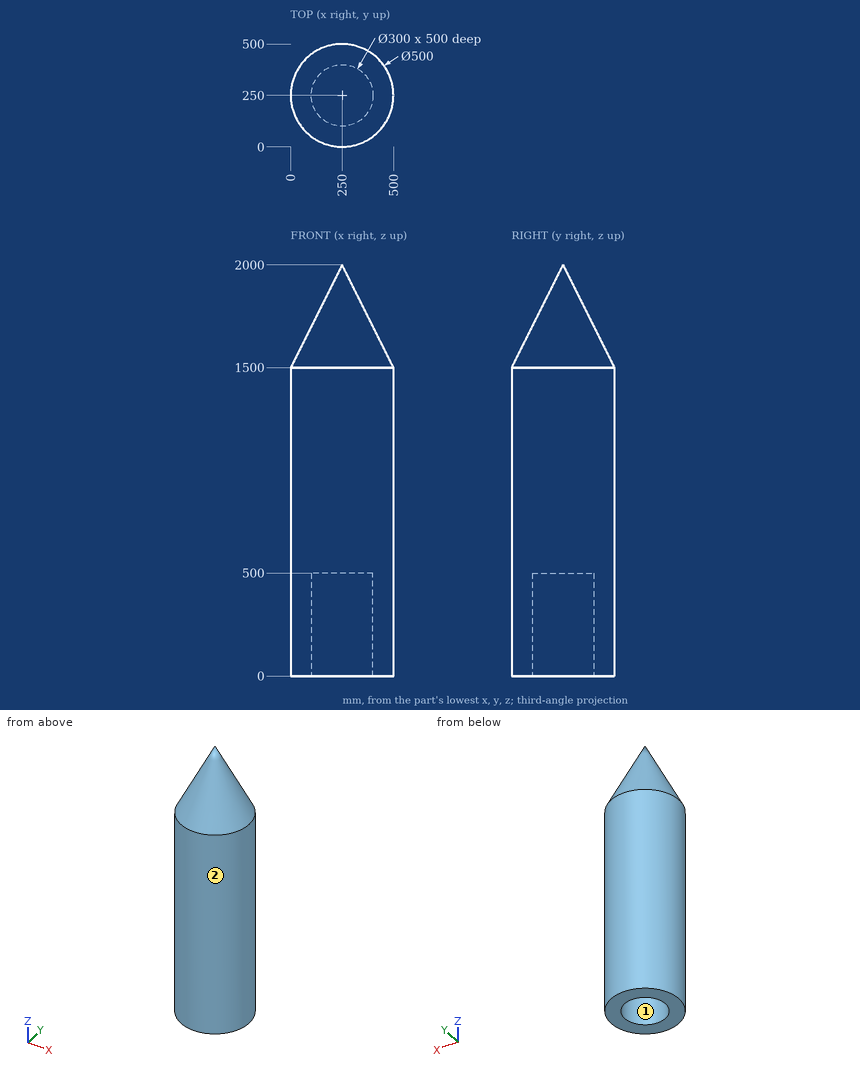
Check sheet for the drawn part. Datum: minimum x, y, z corner. Units: mm. A direction names the side the tool comes from. Coordinates: 2 decimals unless noted, no trailing zeros. Answer as a JSON object with one key per item and string values.
1. Depth check by flat-ended pin: P1, Ø10, axis at x = 317.5, z = 1062, coming from the +Y side; P2, Ø4, axis at x = 107.5, y = 271.5, coming from the -Z side; P3, Ø2, axis at x = 67.5, z = 450.5, coming from the +Y side. Enter the tip coordinate at first touch or a pass-through.
Outcome:
{"P1": "y = 492.06", "P2": "z = 500", "P3": "y = 421.92"}
2. Access from +Z, -Z, +X, -X, +Y, -Y to the whole of each face (thin tool, end or side, straight path). Record for the marked faces 1 and 2.
Outcome:
{"face 1": "-Z", "face 2": "+Z, -Z"}
3. Scan lines: L1, parallel to Y at x = 250, z = 321; L2, parallel to X at y = 147, z = 916; L3, parallel to X at y = 404, z = 150. Record each from-to range of solid material in increasing order. Write a range as from..to.
Outcome:
{"L1": "0..100, 400..500", "L2": "22.2..477.8", "L3": "53.06..446.94"}
